Can you work these out from the model? Positions are in its coordinate system, mm. Face numbers are marked on the shaded views. A direction names the side the tool comes from. Coordinates: 2 decimals unless noted, no trailing zeros. Return JSON: item names as keys, results as strings. Group by question number.
```python
from build123d import *

# Parameters (mm, degrees)
F1_DEPTH = 25


with BuildPart() as f1:
    # F0 (on Top) → F1 (new body)
    with BuildSketch(Plane.XY):
        with BuildLine():
            Line((50, 85), (-55, 85))
            Line((-55, 85), (-55, 78.25))
            ThreePointArc((-55, 78.25), (-54.707107, 77.542893), (-54, 77.25))
            Line((-54, 77.25), (-52.384848, 77.25))
            ThreePointArc((-52.384848, 77.25), (-47.5, 76.5), (-52.384848, 75.75))
            Line((-52.384848, 75.75), (-54, 75.75))
            ThreePointArc((-54, 75.75), (-54.707107, 75.457107), (-55, 74.75))
            Line((-55, 74.75), (-55, 69.75))
            ThreePointArc((-55, 69.75), (-54.707107, 69.042893), (-54, 68.75))
            Line((-54, 68.75), (-52.384848, 68.75))
            ThreePointArc((-52.384848, 68.75), (-47.5, 68), (-52.384848, 67.25))
            Line((-52.384848, 67.25), (-54, 67.25))
            ThreePointArc((-54, 67.25), (-54.707107, 66.957107), (-55, 66.25))
            Line((-55, 66.25), (-55, 61.25))
            ThreePointArc((-55, 61.25), (-54.707107, 60.542893), (-54, 60.25))
            Line((-54, 60.25), (-52.384848, 60.25))
            ThreePointArc((-52.384848, 60.25), (-47.5, 59.5), (-52.384848, 58.75))
            Line((-52.384848, 58.75), (-54, 58.75))
            ThreePointArc((-54, 58.75), (-54.707107, 58.457107), (-55, 57.75))
            Line((-55, 57.75), (-55, 52.75))
            ThreePointArc((-55, 52.75), (-54.707107, 52.042893), (-54, 51.75))
            Line((-54, 51.75), (-52.384848, 51.75))
            ThreePointArc((-52.384848, 51.75), (-47.5, 51), (-52.384848, 50.25))
            Line((-52.384848, 50.25), (-54, 50.25))
            ThreePointArc((-54, 50.25), (-54.707107, 49.957107), (-55, 49.25))
            Line((-55, 49.25), (-55, 44.25))
            ThreePointArc((-55, 44.25), (-54.707107, 43.542893), (-54, 43.25))
            Line((-54, 43.25), (-52.384848, 43.25))
            ThreePointArc((-52.384848, 43.25), (-47.5, 42.5), (-52.384848, 41.75))
            Line((-52.384848, 41.75), (-54, 41.75))
            ThreePointArc((-54, 41.75), (-54.707107, 41.457107), (-55, 40.75))
            Line((-55, 40.75), (-55, 35.75))
            ThreePointArc((-55, 35.75), (-54.707107, 35.042893), (-54, 34.75))
            Line((-54, 34.75), (-52.384848, 34.75))
            ThreePointArc((-52.384848, 34.75), (-47.5, 34), (-52.384848, 33.25))
            Line((-52.384848, 33.25), (-54, 33.25))
            ThreePointArc((-54, 33.25), (-54.707107, 32.957107), (-55, 32.25))
            Line((-55, 32.25), (-55, 27.25))
            ThreePointArc((-55, 27.25), (-54.707107, 26.542893), (-54, 26.25))
            Line((-54, 26.25), (-52.384848, 26.25))
            ThreePointArc((-52.384848, 26.25), (-47.5, 25.5), (-52.384848, 24.75))
            Line((-52.384848, 24.75), (-54, 24.75))
            ThreePointArc((-54, 24.75), (-54.707107, 24.457107), (-55, 23.75))
            Line((-55, 23.75), (-55, 18.75))
            ThreePointArc((-55, 18.75), (-54.707107, 18.042893), (-54, 17.75))
            Line((-54, 17.75), (-52.384848, 17.75))
            ThreePointArc((-52.384848, 17.75), (-47.5, 17), (-52.384848, 16.25))
            Line((-52.384848, 16.25), (-54, 16.25))
            ThreePointArc((-54, 16.25), (-54.707107, 15.957107), (-55, 15.25))
            Line((-55, 15.25), (-55, 10.25))
            ThreePointArc((-55, 10.25), (-54.707107, 9.542893), (-54, 9.25))
            Line((-54, 9.25), (-52.384848, 9.25))
            ThreePointArc((-52.384848, 9.25), (-47.5, 8.5), (-52.384848, 7.75))
            Line((-52.384848, 7.75), (-54, 7.75))
            ThreePointArc((-54, 7.75), (-54.707107, 7.457107), (-55, 6.75))
            Line((-55, 6.75), (-55, 1.75))
            ThreePointArc((-55, 1.75), (-54.707107, 1.042893), (-54, 0.75))
            Line((-54, 0.75), (-52.384848, 0.75))
            ThreePointArc((-52.384848, 0.75), (-47.5, 0), (-52.384848, -0.75))
            Line((-52.384848, -0.75), (-54, -0.75))
            ThreePointArc((-54, -0.75), (-54.707107, -1.042893), (-55, -1.75))
            Line((-55, -1.75), (-55, -6.75))
            ThreePointArc((-55, -6.75), (-54.707107, -7.457107), (-54, -7.75))
            Line((-54, -7.75), (-52.384848, -7.75))
            ThreePointArc((-52.384848, -7.75), (-47.5, -8.5), (-52.384848, -9.25))
            Line((-52.384848, -9.25), (-54, -9.25))
            ThreePointArc((-54, -9.25), (-54.707107, -9.542893), (-55, -10.25))
            Line((-55, -10.25), (-55, -15.25))
            ThreePointArc((-55, -15.25), (-54.707107, -15.957107), (-54, -16.25))
            Line((-54, -16.25), (-52.384848, -16.25))
            ThreePointArc((-52.384848, -16.25), (-47.5, -17), (-52.384848, -17.75))
            Line((-52.384848, -17.75), (-54, -17.75))
            ThreePointArc((-54, -17.75), (-54.707107, -18.042893), (-55, -18.75))
            Line((-55, -18.75), (-55, -23.75))
            ThreePointArc((-55, -23.75), (-54.707107, -24.457107), (-54, -24.75))
            Line((-54, -24.75), (-52.384848, -24.75))
            ThreePointArc((-52.384848, -24.75), (-47.5, -25.5), (-52.384848, -26.25))
            Line((-52.384848, -26.25), (-54, -26.25))
            ThreePointArc((-54, -26.25), (-54.707107, -26.542893), (-55, -27.25))
            Line((-55, -27.25), (-55, -32.25))
            ThreePointArc((-55, -32.25), (-54.707107, -32.957107), (-54, -33.25))
            Line((-54, -33.25), (-52.384848, -33.25))
            ThreePointArc((-52.384848, -33.25), (-47.5, -34), (-52.384848, -34.75))
            Line((-52.384848, -34.75), (-54, -34.75))
            ThreePointArc((-54, -34.75), (-54.707107, -35.042893), (-55, -35.75))
            Line((-55, -35.75), (-55, -40.75))
            ThreePointArc((-55, -40.75), (-54.707107, -41.457107), (-54, -41.75))
            Line((-54, -41.75), (-52.384848, -41.75))
            ThreePointArc((-52.384848, -41.75), (-47.5, -42.5), (-52.384848, -43.25))
            Line((-52.384848, -43.25), (-54, -43.25))
            ThreePointArc((-54, -43.25), (-54.707107, -43.542893), (-55, -44.25))
            Line((-55, -44.25), (-55, -49.25))
            ThreePointArc((-55, -49.25), (-54.707107, -49.957107), (-54, -50.25))
            Line((-54, -50.25), (-52.384848, -50.25))
            ThreePointArc((-52.384848, -50.25), (-47.5, -51), (-52.384848, -51.75))
            Line((-52.384848, -51.75), (-54, -51.75))
            ThreePointArc((-54, -51.75), (-54.707107, -52.042893), (-55, -52.75))
            Line((-55, -52.75), (-55, -57.75))
            ThreePointArc((-55, -57.75), (-54.707107, -58.457107), (-54, -58.75))
            Line((-54, -58.75), (-52.384848, -58.75))
            ThreePointArc((-52.384848, -58.75), (-47.5, -59.5), (-52.384848, -60.25))
            Line((-52.384848, -60.25), (-54, -60.25))
            ThreePointArc((-54, -60.25), (-54.707107, -60.542893), (-55, -61.25))
            Line((-55, -61.25), (-55, -66.25))
            ThreePointArc((-55, -66.25), (-54.707107, -66.957107), (-54, -67.25))
            Line((-54, -67.25), (-52.384848, -67.25))
            ThreePointArc((-52.384848, -67.25), (-47.5, -68), (-52.384848, -68.75))
            Line((-52.384848, -68.75), (-54, -68.75))
            ThreePointArc((-54, -68.75), (-54.707107, -69.042893), (-55, -69.75))
            Line((-55, -69.75), (-55, -74.75))
            ThreePointArc((-55, -74.75), (-54.707107, -75.457107), (-54, -75.75))
            Line((-54, -75.75), (-52.384848, -75.75))
            ThreePointArc((-52.384848, -75.75), (-47.5, -76.5), (-52.384848, -77.25))
            Line((-52.384848, -77.25), (-54, -77.25))
            ThreePointArc((-54, -77.25), (-54.707107, -77.542893), (-55, -78.25))
            Line((-55, -78.25), (-55, -85))
            Line((-55, -85), (50, -85))
            ThreePointArc((50, -85), (53.535534, -83.535534), (55, -80))
            Line((55, -80), (55, 35))
            Line((55, 35), (55, 80))
            ThreePointArc((55, 80), (53.535534, 83.535534), (50, 85))
        make_face()
        with BuildLine():
            Line((60, 85), (50, 85))
            ThreePointArc((50, 85), (53.535534, 83.535534), (55, 80))
            Line((55, 80), (55, 35))
            Line((55, 35), (60, 35))
            ThreePointArc((60, 35), (63.535534, 36.464466), (65, 40))
            Line((65, 40), (65, 80))
            ThreePointArc((65, 80), (63.535534, 83.535534), (60, 85))
        make_face()
    extrude(amount=F1_DEPTH)


solid = f1.part
```
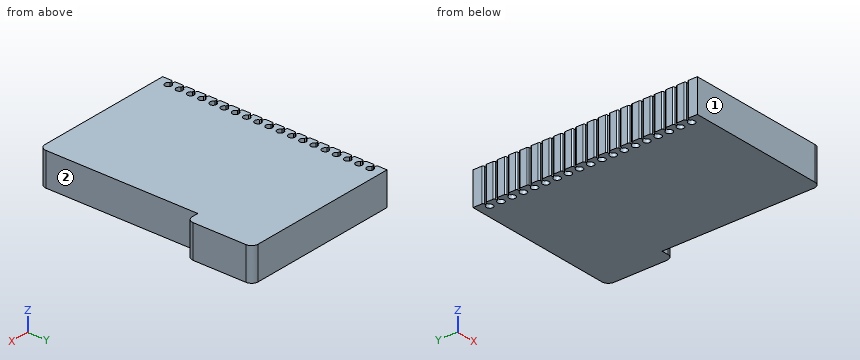
1) If I drill on line 1 (X direction, y = -49.5, z = 22.5); line 2 (X direction, y = 5, z = 22); line 3 (X direction, y = -8, z = 9.75), over which ranges is the centre line in solid material (lowest first)? Write a range as from..to.
2) For the marked faces 1 and 2, which set-ups out of +Z, -Z, +X, -X, +Y, -Y let a thin tool reach every point of the face, with its end or its side?
3) Suppose I cut it at A-A, the plane x = -50. Give the number of separate pieces and of enclosed holes in the cut face, then the cut area to 4 significant figures.
4) For pin 1 (12 mm diameter, centred on y = 30, z = 20, fed in from +X), with a flat end and sliding along its axis, tell me the tip position at first contact or that it passes through.
Returned:
{
 "1": {"line 1": "x = -54.97..-52, -48..55", "line 2": "x = -55..55", "line 3": "x = -47.55..55"},
 "2": {"face 1": "+Z, -Z, +X, -X, -Y", "face 2": "+Z, -Z, +X, -Y"},
 "3": {"separate pieces": "20", "enclosed holes": "0", "area": "1,875 mm²"},
 "4": {"pin 1": "stops at x = 63"}
}
